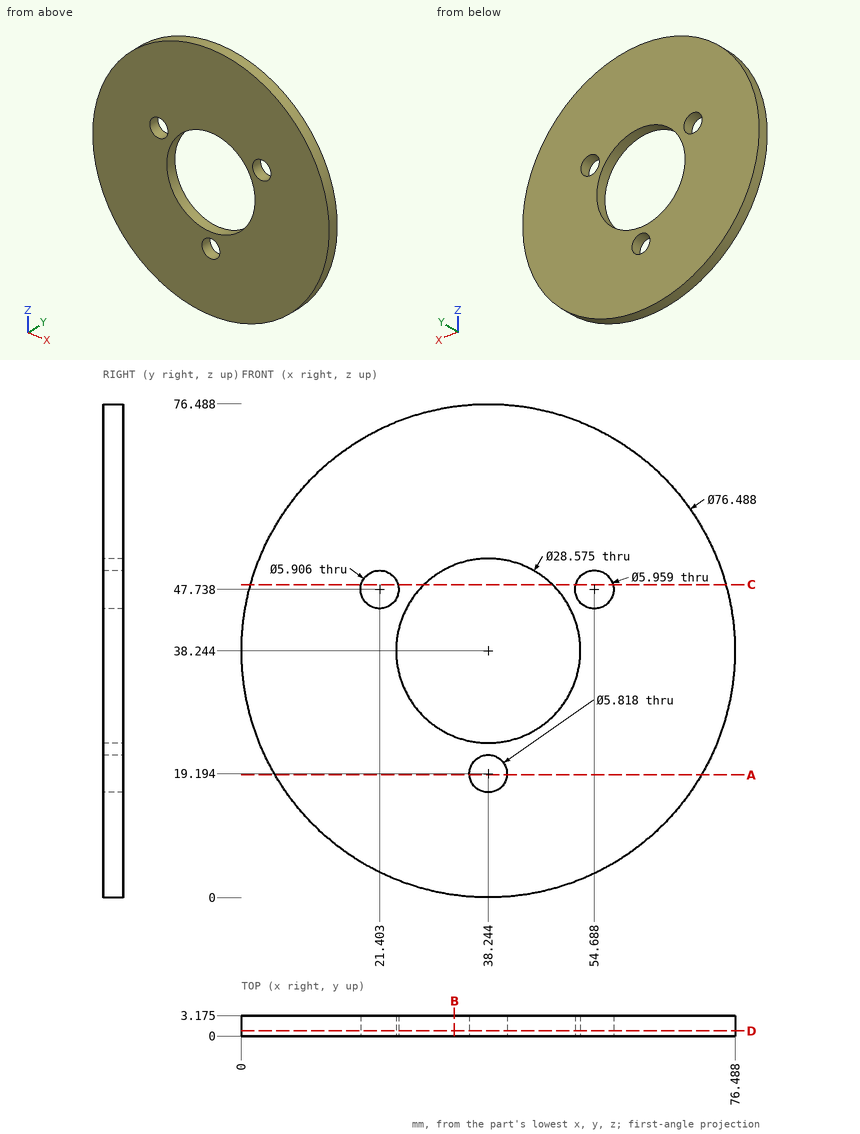
Drawing for the job (mm, zero at the part's lowest x, y, z). Round coordinates to 2 decimals unless told otherwise and drop trailing zeros. Write each loop counter-clockwise with the first axis right and the second up, starting at its lowest first coordinate (ties: lowest second). Pieces come first, ordered by that corner, then holes. Notation, with made-up numbers: (58, -12) - (78, -12) arc R23 cw to (78, 20) - close; hole circle Ø7 at (59, -27). An arc over 180 degrees is marked (long way). Write item = value, one per line. Start each with the question number.
Q1. Band-saw the part on A-A (z = 19). Give the cut face in (x, y) (1 decimal).
Q2. Band-saw the part on B-B (x = 33). Give the cut face in (y, z) (1 decimal).
Q3. Band-saw the part on C-C (z = 48.5). Count the separate pieces of the cut face and the enclosed holes in it, then the cut area to 3 significant figures.
Q4. Probe L1, parallel to Z at x = 37, y = 3 (1 decimal); L2, parallel to Z at x = 32, y = 1.1 (1 decimal); L3, parallel to Z at x = 57, y = 0.9 (1 decimal). List the from-to ranges inside material, lowest first. Write a range as from..to.
Q5. Drop a flat-ended pin along its axis: pin 1 (1.5 mm diameter, centred on x = 25.5, y = 1, fed in from +Z). Give the stop position or say it passes through.
Q6. Band-saw the part on D-D (y = 0.8). Give the cut face in (x, z) (1 decimal), then the cut area to 3 significant figures.
Answers below:
q1.outline = (5.2, 0) - (35.3, 0) - (35.3, 3.2) - (5.2, 3.2) - close; (41.1, 0) - (71.3, 0) - (71.3, 3.2) - (41.1, 3.2) - close
q2.outline = (0, 0.4) - (3.2, 0.4) - (3.2, 25) - (0, 25) - close; (0, 51.5) - (3.2, 51.5) - (3.2, 76.1) - (0, 76.1) - close
q3.separate_pieces = 4
q3.enclosed_holes = 0
q3.area = 134 mm2
q4.L1 = 0..16.6, 21.8..24, 52.5..76.5
q4.L2 = 0.5..25.4, 51.1..76
q4.L3 = 4.9..45.9, 49.6..71.6
q5.pin_1 = 74.56
q6.outline = circle Ø76.5 at (38.2, 38.2); hole circle Ø5.9 at (21.4, 47.7); hole circle Ø28.6 at (38.2, 38.2); hole circle Ø5.8 at (38.2, 19.2); hole circle Ø6 at (54.7, 47.7)
q6.area = 3,870 mm2
